Work out the finished part from the listing and answer in its coordinate system (mm). Face numbers are marked on the shaded views. A direction names the side the tool comes from. Give positions to 0.01 mm unless a question says otherwise; leave off trailing zeros. Write each loop counter-clockwise with the first axis right and the second up, starting at its lowest first coordinate (ties: lowest second). Pieces come first, ordered by that corner, then holes. Notation, with made-up numbers: (5.25, -29.5) -> (15.25, -29.5) arc R30 ccw to (15.25, 3.5) -> close; hole circle Ø9 at (40, -34.75). An arc over 180 degrees is marked (long way). Use a Markdown table: item, result. Add a question column.
Q1. Consider line 1 (Y direction, x = -5, z = 1.25); line 2 (X direction, y = 11.5, z = -2.75); line 3 (Z direction, x = -1.25, y = 75). Determine where each line is inside the solid, lowest interval first.
Q2. For a pull along Y with two mould halves and no side action, classify the marked faces 1 and 2 as pulls with the +Y half, pulls with the -Y half, needs draft (parallel to the pull), parting line crosses it, or undercut.
Q3. For the marked faces 3 and 4, determine the directions among +Z, -Z, +X, -X, +Y, -Y from which every point of the face is accessible in a straight line to the end or side of a thin tool.
Q4. Each of these flat-tipped pins is pushed along its axis until it touches: pin 1 Ø1 at (x, y) = (1.5, 37.5) entering from +Z; pin 2 Ø2 at (x, y) = (4, 23.5) entering from +Z. Where does it stop, or does it pass through?
Q5. Section A-A, the plane y = 6 is taken. Give the vertices of the cut face in (x, z) (3 decimals), plus the area to 3 significant figures.
from build123d import *

# Parameters (mm, degrees)
POCKET_DEPTH = 82.551


with BuildPart() as part:
    # Sketch → Revolution (revolve)
    with BuildSketch(Plane.YZ):
        Polygon((0, 0), (82.55, 0), (82.55, -5.461), (70.326414, -5.461), (69.85, -3.683), (60.325, -3.683), (59.848586, -5.461), (54.451414, -5.461), (53.975, -3.683), (44.45, -3.683), (43.973586, -5.461), (38.576414, -5.461), (38.1, -3.683), (28.575, -3.683), (28.098586, -5.461), (22.701414, -5.461), (22.225, -3.683), (12.7, -3.683), (12.223586, -5.461), (0, -5.461), align=None)
    revolve(axis=Axis((0, 0, 0), (0, 1, 0)))

    # Sketch002 → Pocket (cut, through all)
    with BuildSketch(Plane.XZ):
        with BuildLine():
            ThreePointArc((-1.135923, 2.413), (-2.667, 0), (-1.135923, -2.413))
            Line((-1.135923, -2.413), (-1.135923, -2.964845))
            ThreePointArc((-1.135923, -2.964845), (1.330891, -2.882595), (2.993419, -1.058333))
            Line((2.514472, -0.889), (2.993419, -1.058333))
            ThreePointArc((2.514472, -0.889), (2.667, 0), (2.514472, 0.889))
            Line((2.993419, 1.058333), (2.514472, 0.889))
            ThreePointArc((2.993419, 1.058333), (1.330891, 2.882595), (-1.135923, 2.964845))
            Line((-1.135923, 2.964845), (-1.135923, 2.413))
        make_face()
    extrude(amount=-POCKET_DEPTH, mode=Mode.SUBTRACT)


solid = part.part
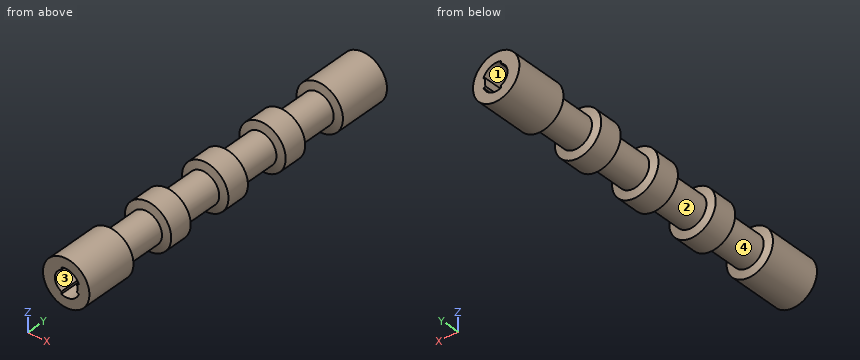
Result set:
| question | item | result |
|---|---|---|
| 1 | line 1 | y = 0 to 12.31, 22.62 to 28.18, 38.49 to 44.06, 54.37 to 59.93, 70.24 to 82.55 |
| 1 | line 2 | x = -4.72 to -1.14, 1.59 to 4.72 |
| 1 | line 3 | z = -5.32 to -2.36, 2.36 to 5.32 |
| 2 | face 1 | needs draft |
| 2 | face 2 | undercut |
| 3 | face 3 | +Y, -Y |
| 3 | face 4 | none |
| 4 | pin 1 | stops at z = 3.54 |
| 4 | pin 2 | stops at z = 4.56 |
| 5 | outline | circle Ø10.922 at (0, 0); hole (-1.136, -2.965) arc R3.175 ccw to (2.993, -1.058) -> (2.514, -0.889) arc R2.667 ccw to (2.514, 0.889) -> (2.993, 1.058) arc R3.175 ccw to (-1.136, 2.965) -> (-1.136, 2.413) arc R2.667 ccw to (-1.136, -2.413) -> close |
| 5 | area | 66.5 mm2 |
